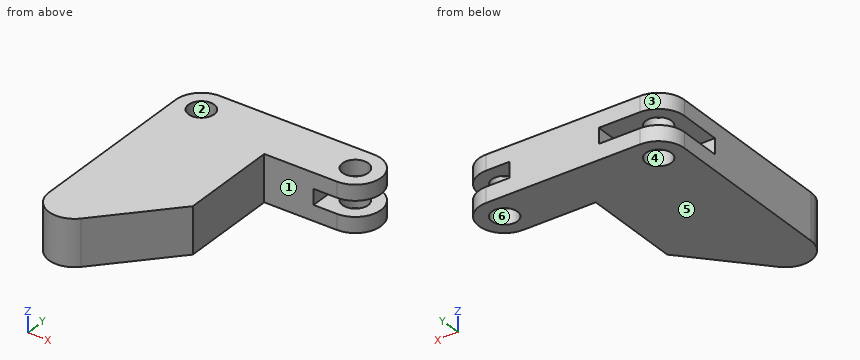
```python
from build123d import *

# Parameters (mm, degrees)
SKETCH1_R           = 2.5
BOSS_EXTRUDE1_DEPTH = 4.5
CUT_EXTRUDE1_DEPTH  = 1.5
CUT_EXTRUDE2_DEPTH  = 1.5
CUT_EXTRUDE3_DEPTH  = 1.5


with BuildPart() as part:
    # Sketch1 → Boss-Extrude1 (new, symmetric)
    with BuildSketch(Plane.XY):
        with BuildLine():
            Line((15, 5), (-15, 5))
            ThreePointArc((-15, 5), (-18.535533906, 3.535533906), (-20, 0))
            Line((-20, 0), (-20, -34.242134344))
            ThreePointArc((-20, -34.242134344), (-16.808430712, -38.903633927), (-11.308168657, -37.614133948))
            Line((-11.308168657, -37.614133948), (0.85432415, -24.298037441))
            Line((0.85432415, -24.298037441), (0.85432415, -5))
            Line((0.85432415, -5), (15, -5))
            ThreePointArc((15, -5), (20, 0), (15, 5))
        make_face()
        with Locations((-15, 0)):
            Circle(SKETCH1_R, mode=Mode.SUBTRACT)
        with Locations((15, 0)):
            Circle(SKETCH1_R, mode=Mode.SUBTRACT)
    extrude(amount=BOSS_EXTRUDE1_DEPTH, both=True)

    # Sketch2 → Cut-Extrude1 (cut, symmetric)
    with BuildSketch(Plane.XY):
        Polygon((-15, 5), (-6.942314992, 5), (-6.942314992, -8.265165355), (-20, -8.265165355), (-20, 0), align=None)
    extrude(amount=CUT_EXTRUDE1_DEPTH, both=True, mode=Mode.SUBTRACT)

    # Sketch4 → Cut-Extrude2 (cut, symmetric)
    with BuildSketch(Plane.XY):
        with BuildLine():
            Line((-20, 0), (-15, 5))
            ThreePointArc((-15, 5), (-18.535533906, 3.535533906), (-20, 0))
        make_face()
    extrude(amount=CUT_EXTRUDE2_DEPTH, both=True, mode=Mode.SUBTRACT)

    # Sketch5 → Cut-Extrude3 (cut, symmetric)
    with BuildSketch(Plane.XY):
        with BuildLine():
            Line((10.468699528, 5), (10.468699528, -5))
            Line((10.468699528, -5), (15, -5))
            ThreePointArc((15, -5), (20, 0), (15, 5))
            Line((15, 5), (10.468699528, 5))
        make_face()
    extrude(amount=CUT_EXTRUDE3_DEPTH, both=True, mode=Mode.SUBTRACT)


solid = part.part
```
Geometry: final body of the model. Coordinates: model frame, mm. Face numbers are marked on the shaded views. A direction names the side the tool comes from. Coordinates: 2 decimals unless noted, no trailing zeros. Order: outer loops, then holes, each group sorted by start corner. A loop starts at its lowest first (then second) coordinate and runs counter-clockwise, first axis right, second up. Notation, with made-up numbers: (-10.5, 53.25) - (45.5, 53.25) arc R16 ccw to (45.5, 75.25) - close; hole circle Ø2 at (-8.5, -37.75). An arc over 180 degrees is marked (long way). Write each question's results on one line, items separated by ' | '.
1) Section D-D, the plane x = 4.5. Return loops of the section in (y, z).
Results list:
outline: (-5, -4.5) - (5, -4.5) - (5, 4.5) - (-5, 4.5) - close
2) Section A-A, the plane z = -3. Return loops of the section in (x, y), plus the area to 3 significant figures.
Results list:
outline: (-20, -34.24) arc R5 ccw to (-11.31, -37.61) - (0.85, -24.3) - (0.85, -5) - (15, -5) arc R5 ccw to (15, 5) - (-15, 5) arc R5 ccw to (-20, 0) - close; hole circle Ø5 at (-15, 0); hole circle Ø5 at (15, 0) | area: 951 mm^2
3) Section B-B, the plane y = -3. Return loops of the section in (x, z), plus the area to 3 significant figures.
Results list:
outline: (-20, -4.5) - (19, -4.5) - (19, -1.5) - (10.47, -1.5) - (10.47, 1.5) - (19, 1.5) - (19, 4.5) - (-20, 4.5) - (-20, 1.5) - (-6.94, 1.5) - (-6.94, -1.5) - (-20, -1.5) - close | area: 286 mm^2
4) Section C-C, the plane x = -13.5. Return loops of the section in (y, z), plus the area to 3 significant figures.
Results list:
outline: (-39.01, -4.5) - (-2, -4.5) - (-2, -1.5) - (-8.27, -1.5) - (-8.27, 1.5) - (-2, 1.5) - (-2, 4.5) - (-39.01, 4.5) - close; (2, -4.5) - (5, -4.5) - (5, -1.5) - (2, -1.5) - close; (2, 1.5) - (5, 1.5) - (5, 4.5) - (2, 4.5) - close | area: 332 mm^2
5) Pull-direction query (X, two-part tool) for the marked faces 3, 4, 5 and 6; classes: pulls with the +X half, pulls with the -X half, needs draft (parallel to the pull), parting line crosses it, or undercut.
Results list:
face 3: pulls with the -X half | face 4: undercut | face 5: needs draft | face 6: undercut
6) Line query: line 1 (X direction, y = 0, z = -3.3); line 2 (Y direction, x = -15, z = 3.65); line 3 (Z direction, x = -15, y = -7). Output: solid intervals per line, ascending. Write a range as from..to.
Results list:
line 1: -20..-17.5, -12.5..12.5, 17.5..20 | line 2: -39.24..-2.5, 2.5..5 | line 3: -4.5..-1.5, 1.5..4.5
7) Pin query (flat end, axial travel): pin 1 (0.9 mm diameter, centred on y = 1, z = 0.5, fed in from +X); pin 2 (5 mm diameter, centred on x = -1, z = -0.5, fed in from -Y); pin 3 (0.9 mm diameter, centred on x = -13, z = 0, fed in from +Y). Return the tip coordinate at first contact, or that it passes through.
Results list:
pin 1: x = 10.47 | pin 2: y = -29.07 | pin 3: y = -8.27
8) Set-up query: the marked faces 1 and 2. Return all of +Z, -Z, +X, -X, +Y, -Y with unobstructed straight access to the full face (end or side cutting, diameter ignored); none if empty.
Results list:
face 1: +Z, -Z, +X, -Y | face 2: +Z, -Z
